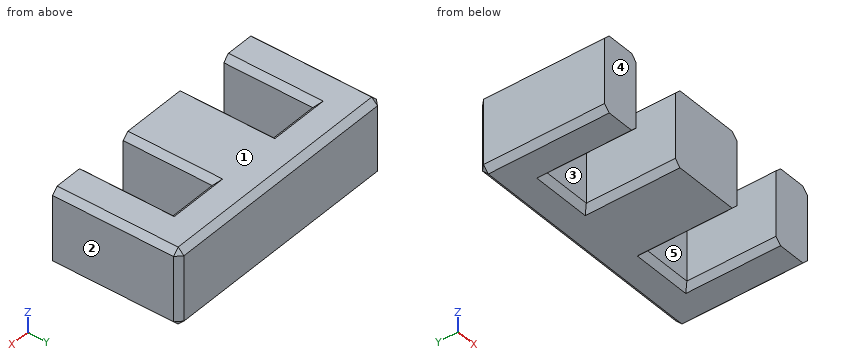
from build123d import *

# Parameters (mm, degrees)
BOSS_EXTRUDE1_DEPTH = 13.2
CHAMFER1_SIZE       = 2


with BuildPart() as part:
    # Sketch1 → Boss-Extrude1 (new, symmetric)
    with BuildSketch(Plane.XY):
        Polygon((43.25, 31.173529412), (-43.25, 31.173529412), (-43.25, -12.426470588), (-29.75, -12.426470588), (-29.75, 18.173529412), (-13.1, 18.173529412), (-13.1, -12.426470588), (13.1, -12.426470588), (13.1, 18.173529412), (29.75, 18.173529412), (29.75, -12.426470588), (43.25, -12.426470588), align=None)
    extrude(amount=BOSS_EXTRUDE1_DEPTH, both=True)

    # Chamfer1
    chamfer1_edges = [part.edges().sort_by_distance(p)[0] for p in [
        (13.1, 2.873529412, -13.2),
        (-13.1, 2.873529412, -13.2),
        (-21.425, 18.173529412, -13.2),
        (-29.75, 2.873529412, -13.2),
        (-43.25, 9.373529412, -13.2),
        (0, 31.173529412, -13.2),
        (43.25, 9.373529412, -13.2),
        (29.75, 2.873529412, -13.2),
        (21.425, 18.173529412, -13.2),
        (43.25, 9.373529412, 13.2),
        (0, 31.173529412, 13.2),
        (-43.25, 31.173529412, 0),
        (43.25, 31.173529412, 0),
        (-43.25, 9.373529412, 13.2),
        (-29.75, 2.873529412, 13.2),
        (-21.425, 18.173529412, 13.2),
        (-13.1, 2.873529412, 13.2),
        (13.1, 2.873529412, 13.2),
        (21.425, 18.173529412, 13.2),
        (29.75, 2.873529412, 13.2),
    ]]
    chamfer(chamfer1_edges, length=CHAMFER1_SIZE)


solid = part.part
Can you work these out from the model? Positions are in its coordinate system, mm. Face numbers are marked on the shaded views. A direction names the side the tool comes from. Give positions to 0.01 mm unless a question says otherwise; leave off trailing zeros. Order: outer loops, then holes, each group sorted by start corner. A loop starts at its lowest first (then second) coordinate and runs counter-clockwise, first axis right, second up. Notation, with made-up numbers: M 73.25,10 L 116.25,10 A16 ccw 116.25,22 Z; hole C -23.5,72 d2. An arc over 180 degrees is marked long. One line per item, written item: value.
Item 1: For the marked faces 4 and 5, which set-ups out of +Z, -Z, +X, -X, +Y, -Y let a thin tool reach every point of the face, with its end or its side?
Verdict:
face 4: +Z, -Z, +X, -X, -Y
face 5: +Z, -Z, -Y
Item 2: For pin 1 (5 mm diameter, centred on x = -19.5, z = 4.5, fed in from -Y); pin 2 (10 mm diameter, centred on x = 28, z = -8.5, fed in from -Y); pin 3 (3 mm diameter, centred on x = 29, y = -1, fed in from +Z), each with a flat end and sliding along its axis, tell me the tip position at first contact or that it passes through.
Verdict:
pin 1: y = 18.17
pin 2: y = -12.43
pin 3: z = 11.95
Item 3: If we section it at C-C on z = -9: Write out the boundary of the cut face in (x, y).
Verdict:
outline: M -43.25,-12.43 L -29.75,-12.43 L -29.75,18.17 L -13.1,18.17 L -13.1,-12.43 L 13.1,-12.43 L 13.1,18.17 L 29.75,18.17 L 29.75,-12.43 L 43.25,-12.43 L 43.25,29.17 L 41.25,31.17 L -41.25,31.17 L -43.25,29.17 Z
Item 4: If we mould it in two halves opening along X, with no side actions, what happens to the marked faces 1, 2 and 3? For each: pulls with the +X half, pulls with the -X half, needs draft (parallel to the pull), parting line crosses it, or undercut.
Verdict:
face 1: needs draft
face 2: pulls with the +X half
face 3: undercut
Item 5: Please list where these lines run through material, in increasing order: line 1 (X direction, y = 4, z = 6.5); line 2 (X direction, y = 7, z = 11.5); line 3 (Y direction, x = 21, z = -4.5).
Verdict:
line 1: -43.25 to -29.75, -13.1 to 13.1, 29.75 to 43.25
line 2: -42.95 to -30.05, -12.8 to 12.8, 30.05 to 42.95
line 3: 18.17 to 31.17
Item 6: If we section it at A-A on y = 7.5: Write out the boundary of the cut face in (x, z), and give its area (3 significant figures).
Verdict:
outline: M -43.25,-11.2 L -41.25,-13.2 L -31.75,-13.2 L -29.75,-11.2 L -29.75,11.2 L -31.75,13.2 L -41.25,13.2 L -43.25,11.2 Z; M -13.1,-11.2 L -11.1,-13.2 L 11.1,-13.2 L 13.1,-11.2 L 13.1,11.2 L 11.1,13.2 L -11.1,13.2 L -13.1,11.2 Z; M 29.75,-11.2 L 31.75,-13.2 L 41.25,-13.2 L 43.25,-11.2 L 43.25,11.2 L 41.25,13.2 L 31.75,13.2 L 29.75,11.2 Z
area: 1,380 mm2
Item 7: If we section it at B-B on x = 23: Write out the boundary of the cut face in (y, z), and give its area (3 significant figures).
Verdict:
outline: M 18.17,-11.2 L 20.17,-13.2 L 29.17,-13.2 L 31.17,-11.2 L 31.17,11.2 L 29.17,13.2 L 20.17,13.2 L 18.17,11.2 Z
area: 335 mm2
